```python
from build123d import *

# Parameters (mm, degrees)
F0_R     = 12.7
F1_DEPTH = 584.2
F2_R     = 9.525
F3_DEPTH = 584.201


# Not quite as in the source:
# - a fillet or chamfer that OpenCascade refuses, or shapes differently, is made with other operations: its cross-section is extruded or revolved along the edge and cut away or added


with BuildPart() as f1:
    # F0 (on Front) → F1 (new body)
    with BuildSketch(Plane.XZ):
        Circle(F0_R)
    extrude(amount=F1_DEPTH)

    # F2 (on face) → F3 (cut, through all)
    with BuildSketch(Plane.XZ.offset(584.2)):
        Circle(F2_R)
    extrude(amount=-F3_DEPTH, mode=Mode.SUBTRACT)

    # F4: fillet of radius 5.08 on 2 edges, made by hand

    # F4_s1 → F4_t2 (revolve, cut)
    with BuildSketch(Plane.XY):
        with BuildLine():
            ThreePointArc((12.7, -579.4907139607), (11.8321134838, -582.3305202921), (9.525, -584.2))
            Line((9.525, -584.2), (12.7, -584.2))
            Line((12.7, -584.2), (12.7, -579.4907139607))
        make_face()
    revolve(axis=Axis((0, -584.2, 0), (0, -1, 0)), mode=Mode.SUBTRACT)

    # F4_s3 → F4_t4 (revolve, cut)
    with BuildSketch(Plane.XY):
        with BuildLine():
            ThreePointArc((12.7, -4.7092860393), (11.8321134838, -1.8694797079), (9.525, 0))
            Line((9.525, 0), (12.7, 0))
            Line((12.7, 0), (12.7, -4.7092860393))
        make_face()
    revolve(axis=Axis((0, 0, 0), (0, -1, 0)), mode=Mode.SUBTRACT)


solid = f1.part
```
Part model, mm, in its own coordinate system. Coordinates: 2 decimals unless noted, no trailing zeros. Order: outer loops, then holes, each group sorted by start corner. A loop starts at its lowest first (then second) coordinate and runs counter-clockwise, first axis right, second up. Notation, with made-up numbers: (48.25, -0.5) - (107.25, -0.5) arc R25 ccw to (107.25, 24.5) - close; hole circle Ø8 at (62.25, 81.25). An arc over 180 degrees is marked (long way). Return JSON: item names as keys, results as strings. Group by question number.
Item 1: Drill centre lines: probe 1 along Z at (x, y) = (0, -430) (3 decimals); probe 2 along Z at (x, y) = (-1.25, -64); probe 3 along X at (y, z) = (-74, 0.25). Where is each one in solid material? Low to high. Write a range as from..to.
Item 2: Cut at A-A (z = 0). List the corners of the cut face in (x, y) (3 decimals), plus the area to 3 significant figures.
Item 3: Pull direction X, two halves, no side cores. Call faces 1 (the face through (-7.559, -296.189, -5.796)), 2 (the face through (-2.75, -288.08, -12.4)): pulls with the +X half, pulls with the -X half, needs draft (parallel to the pull), parting line crosses it, or undercut.
Item 4: Pin check, flat tips, straight feed: pin 1 (1 mm diameter, centred on y = -245.5, z = -6, fed in from +X); pin 2 (1.5 mm diameter, centred on y = -307, z = 3, fed in from +X); pin 3 (5 mm diameter, centred on y = -66, z = -4, fed in from -X); pin 4 (1 mm diameter, centred on x = 8.5, z = 2.5, fed in from +Y). Stop position of each tip, or through.
Item 5: Cut at B-B (x = 0). List the corners of the cut face in (y, z) (3 decimals).
Item 6: Cut at C-C (y = -278). List the corners of the cut face in (x, z) (3 decimals), plus the area to 3 significant figures.
Check values:
{
 "1": {"probe 1": "z = -12.7..-9.525, 9.525..12.7", "probe 2": "z = -12.64..-9.44, 9.44..12.64", "probe 3": "x = -12.7..-9.52, 9.52..12.7"},
 "2": {"outline": "(-12.7, -579.491) arc R5.08 ccw to (-9.525, -584.2) - (-9.525, 0) arc R5.08 ccw to (-12.7, -4.709) - close; (9.525, -584.2) arc R5.08 ccw to (12.7, -579.491) - (12.7, -4.709) arc R5.08 ccw to (9.525, 0) - close", "area": "3,690 mm2"},
 "3": {"face 1": "undercut", "face 2": "parting line crosses it"},
 "4": {"pin 1": "stops at x = 11.45", "pin 2": "stops at x = 12.5", "pin 3": "stops at x = -12.61", "pin 4": "passes through"},
 "5": {"outline": "(-584.2, -9.525) arc R5.08 ccw to (-579.491, -12.7) - (-4.709, -12.7) arc R5.08 ccw to (0, -9.525) - close; (-584.2, 9.525) - (0, 9.525) arc R5.08 ccw to (-4.709, 12.7) - (-579.491, 12.7) arc R5.08 ccw to start"},
 "6": {"outline": "circle Ø25.4 at (0, 0); hole circle Ø19.05 at (0, 0)", "area": "222 mm2"}
}
